from build123d import *

# Parameters (mm, degrees)
SKETCH1_W           = 101.6
SKETCH1_H           = 101.6
BOSS_EXTRUDE1_DEPTH = 9.525
SKETCH2_OUTSIDE_W   = 132.4
SKETCH2_OUTSIDE_H   = 132.4
SKETCH2_OUTSIDE_W_2 = 94.996
SKETCH2_OUTSIDE_H_2 = 94.996
CUT_EXTRUDE1_DEPTH  = 3.175
CHAMFER1_SIZE       = 3.175
CUT_EXTRUDE2_REACH  = 74.471
SKETCH3_R           = 3.175


with BuildPart() as part:
    # Sketch1 → Boss-Extrude1 (new body)
    with BuildSketch(Plane(origin=(0, 0, 0), x_dir=(1, 0, 0), z_dir=(0, 1, 0))):
        Rectangle(SKETCH1_W, SKETCH1_H)
    extrude(amount=BOSS_EXTRUDE1_DEPTH)

    # Sketch2 outside → Cut-Extrude1 (cut)
    with BuildSketch(Plane(origin=(0, 9.525, 0), x_dir=(1, 0, 0), z_dir=(0, 1, 0))):
        Rectangle(SKETCH2_OUTSIDE_W, SKETCH2_OUTSIDE_H)
        Rectangle(SKETCH2_OUTSIDE_W_2, SKETCH2_OUTSIDE_H_2, mode=Mode.SUBTRACT)
    extrude(amount=-CUT_EXTRUDE1_DEPTH, mode=Mode.SUBTRACT)

    # Chamfer1
    chamfer1_edges = [part.edges().sort_by_distance(p)[0] for p in [
        (47.498, 9.525, 0),
        (0, 9.525, -47.498),
        (-47.498, 9.525, 0),
        (0, 9.525, 47.498),
    ]]
    chamfer(chamfer1_edges, length=CHAMFER1_SIZE - 0.0001)  # a hair under: the kernel refuses the full size

    # Sketch3 → Cut-Extrude2 (cut, up to next)
    with BuildSketch(Plane(origin=(0, 9.525, 0), x_dir=(1, 0, 0), z_dir=(0, 1, 0)), mode=Mode.PRIVATE) as cut_extrude2_sk1:
        with Locations(Location((0, 38.1, 0), (0, 0, 270))):
            Circle(SKETCH3_R)
    cut_extrude2_tool1 = extrude(cut_extrude2_sk1.sketch, amount=-CUT_EXTRUDE2_REACH, mode=Mode.PRIVATE) & part.part
    # Sketch3 → Cut-Extrude2 (cut, up to next)
    with BuildSketch(Plane(origin=(0, 9.525, 0), x_dir=(1, 0, 0), z_dir=(0, 1, 0)), mode=Mode.PRIVATE) as cut_extrude2_sk2:
        with Locations(Location((32.995567884, 19.05, 0), (0, 0, 270))):
            Circle(SKETCH3_R)
    cut_extrude2_tool2 = extrude(cut_extrude2_sk2.sketch, amount=-CUT_EXTRUDE2_REACH, mode=Mode.PRIVATE) & part.part
    # Sketch3 → Cut-Extrude2 (cut, up to next)
    with BuildSketch(Plane(origin=(0, 9.525, 0), x_dir=(1, 0, 0), z_dir=(0, 1, 0)), mode=Mode.PRIVATE) as cut_extrude2_sk3:
        with Locations(Location((32.995567884, -19.05, 0), (0, 0, 270))):
            Circle(SKETCH3_R)
    cut_extrude2_tool3 = extrude(cut_extrude2_sk3.sketch, amount=-CUT_EXTRUDE2_REACH, mode=Mode.PRIVATE) & part.part
    # Sketch3 → Cut-Extrude2 (cut, up to next)
    with BuildSketch(Plane(origin=(0, 9.525, 0), x_dir=(1, 0, 0), z_dir=(0, 1, 0)), mode=Mode.PRIVATE) as cut_extrude2_sk4:
        with Locations(Location((0, -38.1, 0), (0, 0, 270))):
            Circle(SKETCH3_R)
    cut_extrude2_tool4 = extrude(cut_extrude2_sk4.sketch, amount=-CUT_EXTRUDE2_REACH, mode=Mode.PRIVATE) & part.part
    # Sketch3 → Cut-Extrude2 (cut, up to next)
    with BuildSketch(Plane(origin=(0, 9.525, 0), x_dir=(1, 0, 0), z_dir=(0, 1, 0)), mode=Mode.PRIVATE) as cut_extrude2_sk5:
        with Locations(Location((-32.995567884, -19.05, 0), (0, 0, 270))):
            Circle(SKETCH3_R)
    cut_extrude2_tool5 = extrude(cut_extrude2_sk5.sketch, amount=-CUT_EXTRUDE2_REACH, mode=Mode.PRIVATE) & part.part
    # Sketch3 → Cut-Extrude2 (cut, up to next)
    with BuildSketch(Plane(origin=(0, 9.525, 0), x_dir=(1, 0, 0), z_dir=(0, 1, 0)), mode=Mode.PRIVATE) as cut_extrude2_sk6:
        with Locations(Location((-32.995567884, 19.05, 0), (0, 0, 270))):
            Circle(SKETCH3_R)
    cut_extrude2_tool6 = extrude(cut_extrude2_sk6.sketch, amount=-CUT_EXTRUDE2_REACH, mode=Mode.PRIVATE) & part.part
    # Sketch3 → Cut-Extrude2 (cut, up to next)
    with BuildSketch(Plane(origin=(0, 9.525, 0), x_dir=(1, 0, 0), z_dir=(0, 1, 0)), mode=Mode.PRIVATE) as cut_extrude2_sk7:
        with Locations(Location((22.225, 0, 0), (0, 0, 270))):
            Circle(SKETCH3_R)
    cut_extrude2_tool7 = extrude(cut_extrude2_sk7.sketch, amount=-CUT_EXTRUDE2_REACH, mode=Mode.PRIVATE) & part.part
    # Sketch3 → Cut-Extrude2 (cut, up to next)
    with BuildSketch(Plane(origin=(0, 9.525, 0), x_dir=(1, 0, 0), z_dir=(0, 1, 0)), mode=Mode.PRIVATE) as cut_extrude2_sk8:
        with Locations(Location((11.1125, -19.247414599, 0), (0, 0, 270))):
            Circle(SKETCH3_R)
    cut_extrude2_tool8 = extrude(cut_extrude2_sk8.sketch, amount=-CUT_EXTRUDE2_REACH, mode=Mode.PRIVATE) & part.part
    # Sketch3 → Cut-Extrude2 (cut, up to next)
    with BuildSketch(Plane(origin=(0, 9.525, 0), x_dir=(1, 0, 0), z_dir=(0, 1, 0)), mode=Mode.PRIVATE) as cut_extrude2_sk9:
        with Locations(Location((-11.1125, -19.247414599, 0), (0, 0, 270))):
            Circle(SKETCH3_R)
    cut_extrude2_tool9 = extrude(cut_extrude2_sk9.sketch, amount=-CUT_EXTRUDE2_REACH, mode=Mode.PRIVATE) & part.part
    # Sketch3 → Cut-Extrude2 (cut, up to next)
    with BuildSketch(Plane(origin=(0, 9.525, 0), x_dir=(1, 0, 0), z_dir=(0, 1, 0)), mode=Mode.PRIVATE) as cut_extrude2_sk10:
        with Locations(Location((-22.225, 0, 0), (0, 0, 270))):
            Circle(SKETCH3_R)
    cut_extrude2_tool10 = extrude(cut_extrude2_sk10.sketch, amount=-CUT_EXTRUDE2_REACH, mode=Mode.PRIVATE) & part.part
    # Sketch3 → Cut-Extrude2 (cut, up to next)
    with BuildSketch(Plane(origin=(0, 9.525, 0), x_dir=(1, 0, 0), z_dir=(0, 1, 0)), mode=Mode.PRIVATE) as cut_extrude2_sk11:
        with Locations(Location((-11.1125, 19.247414599, 0), (0, 0, 270))):
            Circle(SKETCH3_R)
    cut_extrude2_tool11 = extrude(cut_extrude2_sk11.sketch, amount=-CUT_EXTRUDE2_REACH, mode=Mode.PRIVATE) & part.part
    # Sketch3 → Cut-Extrude2 (cut, up to next)
    with BuildSketch(Plane(origin=(0, 9.525, 0), x_dir=(1, 0, 0), z_dir=(0, 1, 0)), mode=Mode.PRIVATE) as cut_extrude2_sk12:
        with Locations(Location((11.1125, 19.247414599, 0), (0, 0, 270))):
            Circle(SKETCH3_R)
    cut_extrude2_tool12 = extrude(cut_extrude2_sk12.sketch, amount=-CUT_EXTRUDE2_REACH, mode=Mode.PRIVATE) & part.part
    # Sketch3 → Cut-Extrude2 (cut, up to next)
    with BuildSketch(Plane(origin=(0, 9.525, 0), x_dir=(1, 0, 0), z_dir=(0, 1, 0)), mode=Mode.PRIVATE) as cut_extrude2_sk13:
        with Locations(Location((0, 0, 0), (0, 0, 270))):
            Circle(SKETCH3_R)
    cut_extrude2_tool13 = extrude(cut_extrude2_sk13.sketch, amount=-CUT_EXTRUDE2_REACH, mode=Mode.PRIVATE) & part.part
    add(cut_extrude2_tool1.solids().sort_by_distance((0, 9.525, -38.1))[0], mode=Mode.SUBTRACT)
    add(cut_extrude2_tool2.solids().sort_by_distance((32.995568, 9.525, -19.05))[0], mode=Mode.SUBTRACT)
    add(cut_extrude2_tool3.solids().sort_by_distance((32.995568, 9.525, 19.05))[0], mode=Mode.SUBTRACT)
    add(cut_extrude2_tool4.solids().sort_by_distance((0, 9.525, 38.1))[0], mode=Mode.SUBTRACT)
    add(cut_extrude2_tool5.solids().sort_by_distance((-32.995568, 9.525, 19.05))[0], mode=Mode.SUBTRACT)
    add(cut_extrude2_tool6.solids().sort_by_distance((-32.995568, 9.525, -19.05))[0], mode=Mode.SUBTRACT)
    add(cut_extrude2_tool7.solids().sort_by_distance((22.225, 9.525, 0))[0], mode=Mode.SUBTRACT)
    add(cut_extrude2_tool8.solids().sort_by_distance((11.1125, 9.525, 19.247415))[0], mode=Mode.SUBTRACT)
    add(cut_extrude2_tool9.solids().sort_by_distance((-11.1125, 9.525, 19.247415))[0], mode=Mode.SUBTRACT)
    add(cut_extrude2_tool10.solids().sort_by_distance((-22.225, 9.525, 0))[0], mode=Mode.SUBTRACT)
    add(cut_extrude2_tool11.solids().sort_by_distance((-11.1125, 9.525, -19.247415))[0], mode=Mode.SUBTRACT)
    add(cut_extrude2_tool12.solids().sort_by_distance((11.1125, 9.525, -19.247415))[0], mode=Mode.SUBTRACT)
    add(cut_extrude2_tool13.solids().sort_by_distance((0, 9.525, 0))[0], mode=Mode.SUBTRACT)


solid = part.part
The listing builds one solid part. Answer for the finished solid, in the listing's coordinates (mm). Coordinates: 2 decimals unless noted, no trailing zeros. Answer as CSV lines item,"result".
1. Determine the mould class of faces 1 (the flat face through (-1, 3, -50.8)), 2 (the flat face through (-50.8, 3, 1)), 3 (the cylindrical face through (25.373, 4.829, -0.413)) for opening direction X: +X half, -X half, draft (parallel to the pull), parting line (faces both ways), or undercut.
Computed values:
face 1,"draft"
face 2,"-X half"
face 3,"undercut"
2. Given P1, Ø1, axis at y = 7, z = -4, coming from the +X side, flat-ended and moving along its own axis, determine where the tip first touches the part or whether it passes through.
Computed values:
P1,"stops at x = 47.35"
3. Find section B-B (z = 0). Give the number of separate pieces and of enclosed holes in the cut face, plus the area to 3 significant figures.
Computed values:
separate pieces,"4"
enclosed holes,"0"
area,"755 mm²"
4. Straight lines are drawn through the part: line 1 (X direction, y = 1, z = 0) (3 decimals); line 2 (X direction, y = 4, z = -19); line 3 (Z direction, x = 10, y = 5.5). For each, find the intervals that lie inside material, in ascending order. Write a range as [from, to].
Computed values:
line 1,"x = [-50.8, -25.4], [-19.05, -3.175], [3.175, 19.05], [25.4, 50.8]"
line 2,"x = [-50.8, -36.17], [-29.82, -14.28], [-7.95, 7.95], [14.28, 29.82], [36.17, 50.8]"
line 3,"z = [-50.8, -22.22], [-16.27, 16.27], [22.22, 50.8]"
